Can you work these out from the model? Positions are in its coordinate system, mm. A direction names the side the tool comes from. Give positions to 0.01 mm unless a question says otherwise; leave off trailing zeros. Order: outer loops, then holes, each group sorted by start corner. A loop starts at its lowest first (then second) coordinate and runs counter-clockwise, first axis right, second up.
```python
from build123d import *

# Parameters (mm, degrees)
EXTRUDE_1_DEPTH          = 6.18
CUT_EXTRUDE_1_DEPTH      = 7.18
FILLET_2_R               = 5
FILLET_3_R               = 5
FILLET_4_R               = 5
FILLET_5_R               = 5
SKETCH_4_W               = 40
SKETCH_4_H               = 6
SKETCH_4_R               = 1.5
CUT_EXTRUDE_2_DEPTH      = 7.18
CUT_EXTRUDE_9_DEPTH      = 1
CUT_EXTRUDE_9_DEPTH_BACK = 7.18


with BuildPart() as part:
    # 草图1 → 凸台-拉伸1 (new body)
    with BuildSketch(Plane(origin=(0, 0, 0), x_dir=(1, 0, 0), z_dir=(0, 1, 0))):
        with BuildLine():
            Line((18.586012984, 33.22179039), (228.586012984, 33.22179039))
            ThreePointArc((228.586012984, 33.22179039), (235.657080796, 30.292858202), (238.586012984, 23.22179039))
            Line((238.586012984, 23.22179039), (238.586012984, -256.77820961))
            ThreePointArc((238.586012984, -256.77820961), (235.657080796, -263.849277422), (228.586012984, -266.77820961))
            Line((228.586012984, -266.77820961), (18.586012984, -266.77820961))
            ThreePointArc((18.586012984, -266.77820961), (11.514945172, -263.849277422), (8.586012984, -256.77820961))
            Line((8.586012984, -256.77820961), (8.586012984, 23.22179039))
            ThreePointArc((8.586012984, 23.22179039), (11.514945172, 30.292858202), (18.586012984, 33.22179039))
        make_face()
    extrude(amount=EXTRUDE_1_DEPTH)

    # 草图2 → 切除-拉伸1 (cut, through all)
    with BuildSketch(Plane(origin=(0, 6.18, 0), x_dir=(1, 0, 0), z_dir=(0, 1, 0))):
        with BuildLine():
            Line((48.586012984, -161.77820961), (48.586012984, -71.77820961))
            ThreePointArc((48.586012984, -71.77820961), (47.12154689, -68.242675704), (43.586012984, -66.77820961))
            Line((43.586012984, -66.77820961), (8.586012984, -66.77820961))
            Line((8.586012984, -66.77820961), (8.586012984, -166.77820961))
            Line((8.586012984, -166.77820961), (43.586012984, -166.77820961))
            ThreePointArc((43.586012984, -166.77820961), (47.12154689, -165.313743516), (48.586012984, -161.77820961))
        make_face()
        with BuildLine():
            Line((56.586012984, -103.77820961), (56.586012984, -108.27820961))
            ThreePointArc((56.586012984, -108.27820961), (55.086012984, -109.77820961), (53.586012984, -108.27820961))
            Line((53.586012984, -108.27820961), (53.586012984, -103.77820961))
            ThreePointArc((53.586012984, -103.77820961), (55.086012984, -102.27820961), (56.586012984, -103.77820961))
        make_face()
        with BuildLine():
            Line((70.586012984, -103.77820961), (70.586012984, -108.27820961))
            ThreePointArc((70.586012984, -108.27820961), (69.086012984, -109.77820961), (67.586012984, -108.27820961))
            Line((67.586012984, -108.27820961), (67.586012984, -103.77820961))
            ThreePointArc((67.586012984, -103.77820961), (69.086012984, -102.27820961), (70.586012984, -103.77820961))
        make_face()
        with BuildLine():
            Line((70.586012984, -129.77820961), (70.586012984, -125.27820961))
            ThreePointArc((70.586012984, -125.27820961), (69.086012984, -123.77820961), (67.586012984, -125.27820961))
            Line((67.586012984, -125.27820961), (67.586012984, -129.77820961))
            ThreePointArc((67.586012984, -129.77820961), (69.086012984, -131.27820961), (70.586012984, -129.77820961))
        make_face()
        with BuildLine():
            Line((56.586012984, -129.77820961), (56.586012984, -125.27820961))
            ThreePointArc((56.586012984, -125.27820961), (55.086012984, -123.77820961), (53.586012984, -125.27820961))
            Line((53.586012984, -125.27820961), (53.586012984, -129.77820961))
            ThreePointArc((53.586012984, -129.77820961), (55.086012984, -131.27820961), (56.586012984, -129.77820961))
        make_face()
        with BuildLine():
            Line((176.586012984, -129.77820961), (176.586012984, -125.27820961))
            ThreePointArc((176.586012984, -125.27820961), (178.086012984, -123.77820961), (179.586012984, -125.27820961))
            Line((179.586012984, -125.27820961), (179.586012984, -129.77820961))
            ThreePointArc((179.586012984, -129.77820961), (178.086012984, -131.27820961), (176.586012984, -129.77820961))
        make_face()
        with BuildLine():
            Line((190.586012984, -129.77820961), (190.586012984, -125.27820961))
            ThreePointArc((190.586012984, -125.27820961), (192.086012984, -123.77820961), (193.586012984, -125.27820961))
            Line((193.586012984, -125.27820961), (193.586012984, -129.77820961))
            ThreePointArc((193.586012984, -129.77820961), (192.086012984, -131.27820961), (190.586012984, -129.77820961))
        make_face()
        with BuildLine():
            Line((190.586012984, -103.77820961), (190.586012984, -108.27820961))
            ThreePointArc((190.586012984, -108.27820961), (192.086012984, -109.77820961), (193.586012984, -108.27820961))
            Line((193.586012984, -108.27820961), (193.586012984, -103.77820961))
            ThreePointArc((193.586012984, -103.77820961), (192.086012984, -102.27820961), (190.586012984, -103.77820961))
        make_face()
        with BuildLine():
            Line((176.586012984, -103.77820961), (176.586012984, -108.27820961))
            ThreePointArc((176.586012984, -108.27820961), (178.086012984, -109.77820961), (179.586012984, -108.27820961))
            Line((179.586012984, -108.27820961), (179.586012984, -103.77820961))
            ThreePointArc((179.586012984, -103.77820961), (178.086012984, -102.27820961), (176.586012984, -103.77820961))
        make_face()
        with BuildLine():
            Line((198.586012984, -161.77820961), (198.586012984, -71.77820961))
            ThreePointArc((198.586012984, -71.77820961), (200.050479078, -68.242675704), (203.586012984, -66.77820961))
            Line((203.586012984, -66.77820961), (238.586012984, -66.77820961))
            Line((238.586012984, -66.77820961), (238.586012984, -166.77820961))
            Line((238.586012984, -166.77820961), (203.586012984, -166.77820961))
            ThreePointArc((203.586012984, -166.77820961), (200.050479078, -165.313743516), (198.586012984, -161.77820961))
        make_face()
    extrude(amount=-CUT_EXTRUDE_1_DEPTH, mode=Mode.SUBTRACT)

    # 圆角2
    fillet_2_edges = [part.edges().sort_by_distance(p)[0] for p in [
        (8.586012984, 3.09, 66.77820961),
    ]]
    fillet(fillet_2_edges, radius=FILLET_2_R)

    # 圆角3
    fillet_3_edges = [part.edges().sort_by_distance(p)[0] for p in [
        (8.586012984, 3.09, 166.77820961),
    ]]
    fillet(fillet_3_edges, radius=FILLET_3_R)

    # 圆角4
    fillet_4_edges = [part.edges().sort_by_distance(p)[0] for p in [
        (238.586012984, 3.09, 166.77820961),
    ]]
    fillet(fillet_4_edges, radius=FILLET_4_R)

    # 圆角5
    fillet_5_edges = [part.edges().sort_by_distance(p)[0] for p in [
        (238.586012984, 3.09, 66.77820961),
    ]]
    fillet(fillet_5_edges, radius=FILLET_5_R)

    # 草图4 → 切除-拉伸2 (cut, through all)
    with BuildSketch(Plane(origin=(0, 0, 0), x_dir=(-1, 0, 0), z_dir=(0, -1, 0))):
        with Locations((-123.586012984, -59.77820961)):
            Rectangle(SKETCH_4_W, SKETCH_4_H)
        with Locations((-123.586012984, -173.77820961)):
            Rectangle(SKETCH_4_W, SKETCH_4_H)
        with Locations((-232.113924071, -35.249657434)):
            Circle(SKETCH_4_R)
        with Locations((-200.838101897, -53.306761785)):
            Circle(SKETCH_4_R)
        with Locations((-232.113924071, -198.306761785)):
            Circle(SKETCH_4_R)
        with Locations((-200.838101897, -180.249657434)):
            Circle(SKETCH_4_R)
        with Locations((-15.058101897, -198.306761785)):
            Circle(SKETCH_4_R)
        with Locations((-46.333924071, -180.249657434)):
            Circle(SKETCH_4_R)
        with Locations((-46.333924071, -53.306761785)):
            Circle(SKETCH_4_R)
        with Locations((-15.058101897, -35.249657434)):
            Circle(SKETCH_4_R)
    extrude(amount=-CUT_EXTRUDE_2_DEPTH, mode=Mode.SUBTRACT)

    # 草图5 → 切除-拉伸9 (cut, two sides)
    with BuildSketch(Plane(origin=(0, 6.18, 0), x_dir=(1, 0, 0), z_dir=(0, 1, 0))) as cut_extrude_9_sk:
        with BuildLine():
            Line((123.586012984, -266.77820961), (23.586012984, -266.77820961))
            ThreePointArc((23.586012984, -266.77820961), (123.586012984, -186.77820961), (223.586012984, -266.77820961))
            Line((223.586012984, -266.77820961), (123.586012984, -266.77820961))
        make_face()
        with BuildLine():
            Line((23.586012984, 33.22179039), (223.586012984, 33.22179039))
            ThreePointArc((223.586012984, 33.22179039), (123.586012984, -46.77820961), (23.586012984, 33.22179039))
        make_face()
    extrude(amount=CUT_EXTRUDE_9_DEPTH, mode=Mode.SUBTRACT)
    extrude(cut_extrude_9_sk.sketch, amount=-CUT_EXTRUDE_9_DEPTH_BACK, mode=Mode.SUBTRACT)


solid = part.part
```
1) If I drill on line 1 (X direction, y = 5.5, z = 126.5); line 2 (Z direction, x = 54, y = 5.5); line 3 (Z direction, x = 201, y = 2), over which ranges is the centre line in solid material (lowest first)?
2) Suppose I cut it at C-C (z = 155.5). Please give me the cut outline in (x, y).
3) I'm going to push flat-ended pins straight in: pin 1 Ø3.5 at (y, z) = (2, 106) entering from +X; pin 2 Ø1.9 at (x, y) = (117, 2) entering from +Z; pin 3 Ø1.3 at (y, z) = (2.5, 128) entering from -X. Where does each tip first touch, or does it pass through?
4) Suppose I cut it at D-D (y = 3). Give the number of separate pieces and of enclosed holes in the cut face, and give its area (3 significant figures).
5) Suppose I cut it at A-A (z = 40.5). Please give me the cut outline in (x, y), and give its area (3 significant figures).
6) Suppose I cut it at B-B (x = 136). Please give me the cut outline in (y, z), and give its area (3 significant figures).
7) We'd pull the mould along Z, two halves only. Please class faces 1 (the face through (29, 3, 66.778)), 2 (the face through (8.586, 3, 20)), 3 (the face through (11.593, 3.047, 263.927)): +Z half, -Z half, draft (parallel to the pull), parting line (faces both ways), or undercut.
8) Which directions (+Z, -Z, +X, -X, +Y, -Y) give clear straight access to the entire face, cutting with the end or side of a thin tool? Please do faces 4 (the face through (103.586, 3, 60)), 5 (the face through (219, 3, 166.778)), 6 (the face through (48.586, 3, 117)), 7 (the face through (11.438, 3.047, -30.215)).
Results:
1. line 1: x = 48.59 to 53.59, 56.59 to 67.59, 70.59 to 176.59, 179.59 to 190.59, 193.59 to 198.59
1. line 2: z = 19.54 to 102.74, 109.31 to 124.24, 130.81 to 214.02
1. line 3: z = 11.46 to 51.82, 54.8 to 67.5, 166.06 to 178.76, 181.74 to 222.1
2. outline: (48.59, 0) - (198.59, 0) - (198.59, 6.18) - (48.59, 6.18) - close
3. pin 1: stops at x = 198.59
3. pin 2: stops at z = 187.06
3. pin 3: stops at x = 48.59
4. separate pieces: 1
4. enclosed holes: 18
4. area: 36,400 mm2
5. outline: (8.59, 0) - (88.26, 0) - (88.26, 6.18) - (8.59, 6.18) - close; (158.91, 0) - (238.59, 0) - (238.59, 6.18) - (158.91, 6.18) - close
5. area: 985 mm2
6. outline: (0, 46.02) - (6.18, 46.02) - (6.18, 56.78) - (0, 56.78) - close; (0, 62.78) - (6.18, 62.78) - (6.18, 170.78) - (0, 170.78) - close; (0, 176.78) - (6.18, 176.78) - (6.18, 187.53) - (0, 187.53) - close
6. area: 800 mm2
7. face 1: undercut
7. face 2: draft
7. face 3: +Z half
8. face 4: +Y, -Y
8. face 5: +X, +Y, -Y
8. face 6: -X, +Y, -Y
8. face 7: -Z, -X, +Y, -Y
